Could you check a few things on this model? Use its own coordinates, in mm. A direction names the side the tool comes from. Coordinates: 2 decimals unless noted, no trailing zeros. Loops run counter-clockwise (first coordinate to the right, second up) from the corner with the lowest first, then second, coordinate; pieces in that order, holes last.
1) Imagine slicing it at B-B on x = -5.25. Please give me the cut outline in (y, z), plus the area to 3 significant figures.
2) Will these pins go through, and if not, where does the flat tip stop? P1, Ø1, axis at y = -3, z = 2.5, coming from the -X side; P2, Ø1.5, axis at x = 2.5, z = 4.5, coming from the -Y side; P3, Ø3, axis at x = -5, z = 2, coming from the +Y side.
3) Thinking about a two-plate mould opening in Y: for faces 1 (the face through (-2.635, -4.984, 2.504)), 2 (the face through (5.213, -2.214, 2.504)), 3 (the face through (3.96, 4.04, 2.5)), 4 (the face through (0.561, -5.616, 2.504)), which applies, released by +Y, released by -Y, zero draft, split by the parting line, or undercut?
4) Imagine slicing it at C-C on z = -0.75. Please give me the cut outline in (x, y), plus the area to 3 significant figures.
5) If I drill on line 1 along Y through (x, z) = (0, -1.15); line 2 along Y through (x, z) = (-5.5, 1.75); line 3 along Z through (x, y) = (0.5, -0.25), over which ranges is the centre line in solid material (lowest first)?
6) Imagine slicing it at D-D on x = -2.25. Please give me the cut outline in (y, z), plus the area to 3 significant figures.
7) Imagine slicing it at A-A on y = 0. Please give me the cut outline in (x, z).
8) For faces 5 (the face through (1.437, 0, 3)), 6 (the face through (-5.1, -2.41, 2.5)), 7 (the face through (5.067, 2.465, 2.504)), 8 (the face through (-0.89, -5.59, 2.5)), which set-ups out of +Z, -Z, +X, -X, +Y, -Y let a thin tool reach every point of the face, with its end or its side?
```python
from build123d import *

# Parameters (mm, degrees)
SKETCH1_R           = 6.35
BOSS_EXTRUDE1_DEPTH = 5.08
SKETCH2_R           = 0.804650072
CUT_EXTRUDE1_DEPTH  = 5.08
CUT_EXTRUDE4_DEPTH  = 5.08
SKETCH7_R           = 3.476857069
BOSS_EXTRUDE3_DEPTH = 2.258601292
SKETCH10_R          = 0.804650072
CUT_EXTRUDE5_DEPTH  = 5.12259779
SKETCH11_R          = 0.474817283
CUT_EXTRUDE6_DEPTH  = 9.144


with BuildPart() as part:
    # Sketch1 → Boss-Extrude1 (new body)
    with BuildSketch(Plane.XY):
        Circle(SKETCH1_R)
    extrude(amount=BOSS_EXTRUDE1_DEPTH)

    # Sketch2 → Cut-Extrude1 (cut)
    with BuildSketch(Plane.XY.offset(5.08)):
        Circle(SKETCH2_R)
    extrude(amount=-CUT_EXTRUDE1_DEPTH, mode=Mode.SUBTRACT)

    # Sketch6 → Cut-Extrude4 (cut)
    with BuildSketch(Plane(origin=(0, 0, 0), x_dir=(-1, 0, 0), z_dir=(0, 0, -1))):
        with BuildLine():
            Line((-6.313419859, 0.680609785), (-4.841727293, 1.082552663))
            ThreePointArc((-4.841727293, 1.082552663), (-4.737782551, 1.472297507), (-4.602520026, 1.852310143))
            Line((-4.602520026, 1.852310143), (-5.544711841, 3.094942746))
            ThreePointArc((-5.544711841, 3.094942746), (-6.050708452, 1.926506484), (-6.313419859, 0.680609785))
        make_face()
        with BuildLine():
            ThreePointArc((-4.621895526, -1.803420416), (-4.697643554, -1.595740734), (-4.764064977, -1.384892901))
            Line((-4.764064977, -1.384892901), (-6.284089397, -0.912535181))
            ThreePointArc((-6.284089397, -0.912535181), (-6.095179755, -1.780809857), (-5.786915427, -2.614213043))
            Line((-5.786915427, -2.614213043), (-4.621895526, -1.803420416))
        make_face()
        with BuildLine():
            ThreePointArc((-2.49633596, -4.287487636), (-2.747933203, -4.130751331), (-2.989720929, -3.959269152))
            Line((-2.989720929, -3.959269152), (-4.414172057, -4.564820375))
            ThreePointArc((-4.414172057, -4.564820375), (-3.704724213, -5.157278207), (-2.916783485, -5.640467543))
            Line((-2.916783485, -5.640467543), (-2.49633596, -4.287487636))
        make_face()
        with BuildLine():
            ThreePointArc((0.658971441, -4.91731635), (0.164985262, -4.958530358), (-0.330647946, -4.950243972))
            Line((-0.330647946, -4.950243972), (-0.797062617, -6.299777074))
            ThreePointArc((-0.797062617, -6.299777074), (0.162157154, -6.347929194), (1.117667403, -6.250865506))
            Line((1.117667403, -6.250865506), (0.658971441, -4.91731635))
        make_face()
        with BuildLine():
            ThreePointArc((3.079848524, -3.889572794), (2.834017843, -4.072172186), (2.577390132, -4.23925743))
            Line((2.577390132, -4.23925743), (2.695058949, -5.74970932))
            ThreePointArc((2.695058949, -5.74970932), (3.630700167, -5.209656063), (4.461255519, -4.518816127))
            Line((4.461255519, -4.518816127), (3.079848524, -3.889572794))
        make_face()
        with BuildLine():
            ThreePointArc((4.764064977, -1.384892901), (4.689120213, -1.620615648), (4.602520026, -1.852310143))
            Line((4.602520026, -1.852310143), (5.609586886, -2.975741079))
            ThreePointArc((5.609586886, -2.975741079), (6.026210342, -2.001821398), (6.2751364, -0.972195025))
            Line((6.2751364, -0.972195025), (4.764064977, -1.384892901))
        make_face()
        with BuildLine():
            ThreePointArc((4.697742855, 1.595448377), (4.785985372, 1.307129477), (4.856550498, 1.013982598))
            Line((4.856550498, 1.013982598), (6.301072583, 0.786755552))
            ThreePointArc((6.301072583, 0.786755552), (6.117140529, 1.703846165), (5.800483524, 2.583968051))
            Line((5.800483524, 2.583968051), (4.697742855, 1.595448377))
        make_face()
        with BuildLine():
            Line((-4.631054346, 4.34463297), (-3.274854363, 3.726871658))
            ThreePointArc((-3.274854363, 3.726871658), (-2.997527533, 3.953362131), (-2.704587495, 4.159260744))
            Line((-2.704587495, 4.159260744), (-2.823654461, 5.68765993))
            ThreePointArc((-2.823654461, 5.68765993), (-3.787360718, 5.096900901), (-4.631054346, 4.34463297))
        make_face()
        with BuildLine():
            Line((-1.15729269, 6.243650665), (-0.330647946, 4.950243972))
            ThreePointArc((-0.330647946, 4.950243972), (0.099169547, 4.960283142), (0.528242314, 4.933072421))
            Line((0.528242314, 4.933072421), (1.127688946, 6.249065341))
            ThreePointArc((1.127688946, 6.249065341), (-0.015047428, 6.349982171), (-1.15729269, 6.243650665))
        make_face()
        with BuildLine():
            Line((2.80655769, 5.696115688), (2.577390132, 4.23925743))
            ThreePointArc((2.577390132, 4.23925743), (2.937316156, 3.998301796), (3.274854363, 3.726871658))
            Line((3.274854363, 3.726871658), (4.557114361, 4.422127169))
            ThreePointArc((4.557114361, 4.422127169), (3.736532912, 5.134279092), (2.80655769, 5.696115688))
        make_face()
    extrude(amount=-CUT_EXTRUDE4_DEPTH, mode=Mode.SUBTRACT)

    # Sketch7 → Boss-Extrude3 (add)
    with BuildSketch(Plane(origin=(0, 0, 0), x_dir=(-1, 0, 0), z_dir=(0, 0, -1))):
        Circle(SKETCH7_R)
    extrude(amount=BOSS_EXTRUDE3_DEPTH)

    # Sketch10 → Cut-Extrude5 (cut)
    with BuildSketch(Plane.XY.offset(5.08)):
        Circle(SKETCH10_R)
        Polygon((1.437219643, 0), (1.437219643, -1.996796237), (1.079397463, -2.210813568), (0.451137939, -2.418526426), (0, -2.460242979), (-0.588709584, -2.388768834), (-1.06538084, -2.217602124), (-1.420507786, -2.008719279), (-1.420507786, 0), (0, 0), align=None)
        with BuildLine():
            Line((-0.804650072, 0), (0, 0))
            Line((0, 0), (0.804650072, 0))
            ThreePointArc((0.804650072, 0), (0, 0.804650072), (-0.804650072, 0))
        make_face()
        with BuildLine():
            Line((0.804650072, 0), (0, 0))
            Line((0, 0), (-0.804650072, 0))
            ThreePointArc((-0.804650072, 0), (0, -0.804650072), (0.804650072, 0))
        make_face()
        Polygon((1.437219643, 1.996796237), (1.437219643, 0), (0, 0), (-1.420507786, 0), (-1.420507786, 2.008719279), (-0.710253893, 2.355490378), (0, 2.460242979), (0.902275879, 2.288819292), align=None)
    extrude(amount=-CUT_EXTRUDE5_DEPTH, mode=Mode.SUBTRACT)

    # Sketch11 → Cut-Extrude6 (cut)
    with BuildSketch(Plane(origin=(0, 0, -2.258601292), x_dir=(-1, 0, 0), z_dir=(0, 0, -1))):
        Circle(SKETCH11_R)
    extrude(amount=-CUT_EXTRUDE6_DEPTH, mode=Mode.SUBTRACT)


solid = part.part
```
Filled in:
1. outline: (-3.57, 0) - (-2.57, 0) - (-2.57, 5.08) - (-3.57, 5.08) - close; (-1.25, 0) - (0.95, 0) - (0.95, 5.08) - (-1.25, 5.08) - close; (2.09, 0) - (3.57, 0) - (3.57, 5.08) - (2.09, 5.08) - close
1. area: 23.8 mm2
2. P1: stops at x = -5.61
2. P2: stops at y = -6.1
2. P3: stops at y = 4.42
3. face 1: undercut
3. face 2: undercut
3. face 3: released by +Y
3. face 4: released by -Y
4. outline: circle Ø6.95 at (0, 0); hole circle Ø0.95 at (0, 0)
4. area: 37.3 mm2
5. line 1: y = -3.48 to -0.47, 0.47 to 3.48
5. line 2: y = -3.17 to -2.85, -1.18 to 0.91, 2.31 to 3.17
5. line 3: z = -2.26 to -0.04
6. outline: (-5.94, 0) - (-2.65, 0) - (-2.65, -2.26) - (2.65, -2.26) - (2.65, 0) - (5.94, 0) - (5.94, 5.08) - (-5.94, 5.08) - close
6. area: 72.3 mm2
7. outline: (-6.35, 0) - (-3.48, 0) - (-3.48, -2.26) - (-0.47, -2.26) - (-0.47, -0.04) - (-1.42, -0.04) - (-1.42, 5.08) - (-6.35, 5.08) - close; (0.47, -2.26) - (3.48, -2.26) - (3.48, 0) - (6.35, 0) - (6.35, 5.08) - (1.44, 5.08) - (1.44, -0.04) - (0.47, -0.04) - close
8. face 5: +Z
8. face 6: +Z, -Z, -X
8. face 7: +Z, -Z, +X
8. face 8: +Z, -Z, -Y
